Source: CAD feature listing. Evaluate the final solid. Frame: model axes, mm. Face numbers are marked on the shaded views. A direction names the side the tool comes from. Give positions to 0.01 mm unless a question says otherwise; leave off trailing zeros. Loops run counter-clockwise (first coordinate to the right, second up) from the corner with the lowest first, then second, coordinate; pieces in that order, holes last. Notation, with made-up numbers: (-11, 52.5) -> (12, 52.5) arc R22 cw to (12, 90.5) -> close; hole circle Ø2 at (-5, -10). An arc over 180 degrees is marked (long way). Put each result on its own line as item: value.
```python
from build123d import *

# Parameters (mm, degrees)
F1_DEPTH = 3.125
F2_R     = 0.6
F3_DEPTH = 5


with BuildPart() as f1:
    # F0 (on Top) → F1 (new body)
    with BuildSketch(Plane.XY):
        Polygon((-7.604167, 6.5625), (-7.604167, 0), (-4.479167, 0), (-4.479167, 3.4375), (0, 3.4375), (0, 6.5625), (-6.604167, 6.5625), align=None)
        Polygon((-9.104167, 13.854167), (-7.604167, 6.5625), (-6.604167, 6.5625), (-5.104167, 13.854167), align=None)
    extrude(amount=F1_DEPTH)

    # F2 (on face) → F3 (cut)
    with BuildSketch(Plane.XZ):
        with Locations((-6.041667, 1.5625)):
            Circle(F2_R)
    extrude(amount=-F3_DEPTH, mode=Mode.SUBTRACT)


solid = f1.part
```
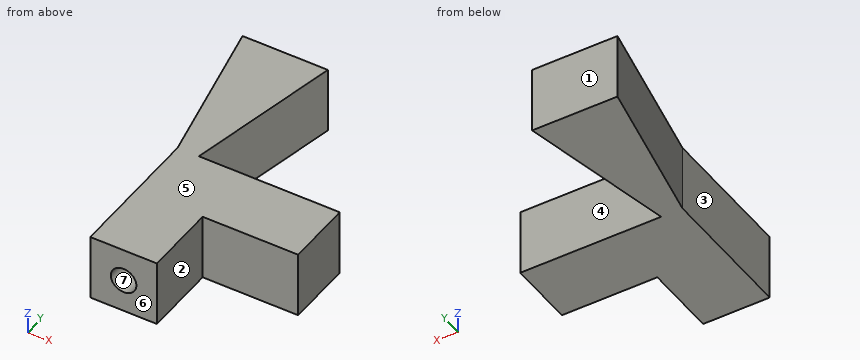
(1) Section A-A on z = 2.85. Return loops of the section in (x, y), then the cut area to 3 significant figures.
Calculated:
outline: (-9.1, 13.85) -> (-7.6, 6.56) -> (-7.6, 0) -> (-4.48, 0) -> (-4.48, 3.44) -> (0, 3.44) -> (0, 6.56) -> (-6.6, 6.56) -> (-5.1, 13.85) -> close
area: 52.7 mm²
(2) First-contact query: P1, Ø5, axis at x = -6, y = 3.5, coming from the -Z side; P2, Ø1.6, axis at x = -2.5, z = 1, coming from the +Y side. Flat tips, straight axial feed; report the tip coordinate or a pass-through.
Calculated:
P1: stops at z = 0
P2: stops at y = 6.56
(3) Section B-B on x = -5.75. Return loops of the section in (y, z) (1 decimal), then the cut area to 3 significant figures.
Calculated:
outline: (0, 0) -> (6.6, 0) -> (6.6, 3.1) -> (0, 3.1) -> (0, 2.1) -> (5, 2.1) -> (5, 1) -> (0, 1) -> close; (10.7, 0) -> (13.9, 0) -> (13.9, 3.1) -> (10.7, 3.1) -> close
area: 25.1 mm²
(4) Section D-D on y = 2.75. Return loops of the section in (x, z) (1 decimal), then the cut area to 3 significant figures.
Calculated:
outline: (-7.6, 0) -> (-4.5, 0) -> (-4.5, 3.1) -> (-7.6, 3.1) -> close; hole circle Ø1.2 at (-6, 1.6)
area: 8.63 mm²
(5) Reachability of the marked faces 1, 2, 3 and 4 from +Z, -Z, +X, -X, +Y, -Y: full face, straight path, thin tool, end or side. Return the list, or none.
Calculated:
face 1: +Z, -Z, +X, -X, +Y
face 2: +Z, -Z, +X, -Y
face 3: +Z, -Z, -X, -Y
face 4: +Z, -Z, +X
(6) Section C-C on x = -1.25. Return loops of the section in (y, z) (1 decimal).
Calculated:
outline: (3.4, 0) -> (6.6, 0) -> (6.6, 3.1) -> (3.4, 3.1) -> close
(7) Draft query along Z for the marked faces 5, 6 and 7. Return one class per face: released by +Z, released by -Z, zero draft, split by the parting line, or undercut.
Calculated:
face 5: released by +Z
face 6: zero draft
face 7: undercut
(8) Line query: probe 1 along Y at (x, z) = (-0.75, 0.25); probe 2 along Z at (x, y) = (-6, 4) (3 decimals); probe 3 along X at (y, z) = (1.75, 2.8). Output: solid intervals per line, ascending. Write a range as from..to.
Calculated:
probe 1: y = 3.44..6.56
probe 2: z = 0..0.964, 2.161..3.125
probe 3: x = -7.6..-4.48
